Study the drawing (mm; zero at the part's minimum x, y, z) and answer. A direction names the side the tool comes from. Round coordinates to 2 decimals unless told otherwise and drop trailing zeros. Write each loop counter-clockwise with the first axis right and the second up, starting at its lowest first coordinate (ties: lowest second). Pieces come first, ordered by that corner, then holes.
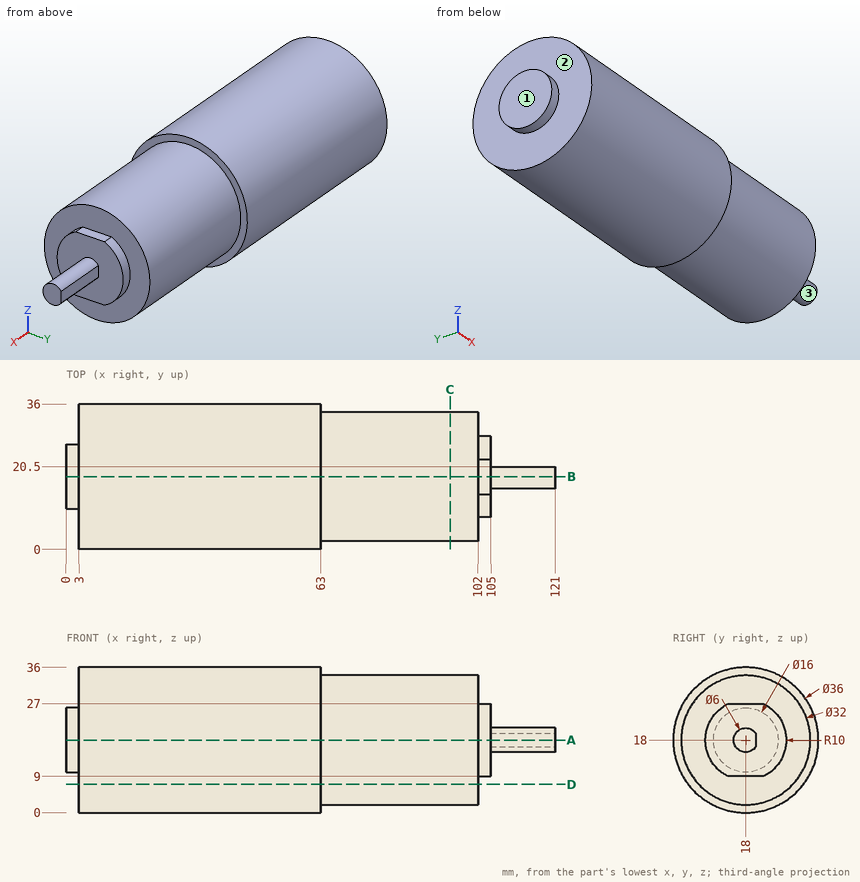
Q1. Find the intervals of material crossed by L1, parallel to X at y = 15, z = 28; L2, parallel to X at y = 10.5, z = 17; L3, parallel to Z at x = 38, y = 25.5, in increasing order.
Q2. Given pin 1 (4 mm diameter, centred on y = 24.5, z = 12, fed in from +X); pin 2 (1.5 mm diameter, centred on x = 85, y = 27, fed in from -Z); pin 3 (2 mm diameter, centred on x = 52.5, z = 21.5, fed in from +Y); pin 4 (2 mm diameter, centred on x = 103.5, z = 31, fed in from +Y), each flat-ended and moving along its own axis, determine where each tip first touches the part or whether it passes through.
Q3. Find section C-C (x = 95). Determine the outline of the cut face in (y, z).
Q4. Find section D-D (z = 7). Determine the outline of the cut face in (x, y), plus the area to 3 significant figures.
Q5. Find section A-A (z = 18). Determine the outline of the cut face in (x, y).
Q6. Find section B-B (y = 18). Determine the outline of the cut face in (x, z).
Q7. A tool of negligible diameter and unlimited length cuts with its end or side. For the marked faces 1, 2 and 3, from which of +Z, -Z, +X, -X, +Y, -Y can it reach the whole face along a straight path? Write none if from no direction.
Report:
1. L1: x = 3 to 102
1. L2: x = 0 to 105
1. L3: z = 1.64 to 34.36
2. pin 1: stops at x = 105
2. pin 2: stops at z = 4.29
2. pin 3: stops at y = 35.83
2. pin 4: passes through
3. outline: circle Ø32 at (18, 18)
4. outline: (3, 3.75) - (63, 3.75) - (63, 6.38) - (102, 6.38) - (102, 29.62) - (63, 29.62) - (63, 32.25) - (3, 32.25) - close
4. area: 2,620 mm2
5. outline: (0, 10) - (3, 10) - (3, 0) - (63, 0) - (63, 2) - (102, 2) - (102, 8) - (105, 8) - (105, 15) - (121, 15) - (121, 20.5) - (105, 20.5) - (105, 28) - (102, 28) - (102, 34) - (63, 34) - (63, 36) - (3, 36) - (3, 26) - (0, 26) - close
6. outline: (0, 10) - (3, 10) - (3, 0) - (63, 0) - (63, 2) - (102, 2) - (102, 9) - (105, 9) - (105, 15) - (121, 15) - (121, 21) - (105, 21) - (105, 27) - (102, 27) - (102, 34) - (63, 34) - (63, 36) - (3, 36) - (3, 26) - (0, 26) - close
7. face 1: +Z, -Z, -X, +Y, -Y
7. face 2: -X
7. face 3: +X
